```python
from build123d import *

# Parameters (mm, degrees)
F1_DEPTH = 3.175
F2_R     = 5.08
F3_R     = 5.08


with BuildPart() as f1:
    # F0 (on Front) → F1 (new body)
    with BuildSketch(Plane.XZ):
        with BuildLine():
            Line((-6.35, 0), (0, 0))
            Line((0, 0), (0, 22.86))
            Line((0, 22.86), (-6.35, 22.86))
            Line((-6.35, 22.86), (-6.35, 19.685))
            ThreePointArc((-6.35, 19.685), (-4.104936, 18.755064), (-3.175, 16.51))
            ThreePointArc((-3.175, 16.51), (-4.104936, 14.264936), (-6.35, 13.335))
            Line((-6.35, 13.335), (-6.35, 0))
        make_face()
        with BuildLine():
            Line((-12.7, 0), (-6.35, 0))
            Line((-6.35, 0), (-6.35, 13.335))
            ThreePointArc((-6.35, 13.335), (-9.525, 16.51), (-6.35, 19.685))
            Line((-6.35, 19.685), (-6.35, 22.86))
            Line((-6.35, 22.86), (-12.7, 22.86))
            Line((-12.7, 22.86), (-12.7, 0))
        make_face()
    extrude(amount=F1_DEPTH)

    # F2
    f2_edges = [f1.edges().sort_by_distance(p)[0] for p in [
        (0, -1.5875, 22.86),
    ]]
    fillet(f2_edges, radius=F2_R)

    # F3
    f3_edges = [f1.edges().sort_by_distance(p)[0] for p in [
        (-12.7, -1.5875, 22.86),
    ]]
    fillet(f3_edges, radius=F3_R)


solid = f1.part
```
CAD build for the part. Positions are in the model's coordinates, mm. Give positions to 0.01 mm unless a question says otherwise; leave off trailing zeros. Order: outer loops, then holes, each group sorted by start corner. A loop starts at its lowest first (then second) coordinate and runs counter-clockwise, first axis right, second up.
(1) Saw through at B-B, the plane x = -5.75. Give the cut face in (y, z) (3 decimals), then the cut area to 3 significant figures.
(2) Saw through at A-A, the plane y = -0.9. Give the cut face in (x, z) (3 decimals), then the cut area to 3 significant figures.
(3) Drill centre lines: L1, parallel to X at y = -0.85, z = 16.5; L2, parallel to Z at x = -8, y = -2.75; L3, parallel to Z at x = -4.75, y = -0.3. Where is each one in solid material? Low to high.
(4) Saw through at C-C, the plane z = 17.25. Give the cut face in (x, y) (3 decimals).
Results found:
1. outline: (-3.175, 0) - (0, 0) - (0, 13.392) - (-3.175, 13.392) - close; (-3.175, 19.628) - (0, 19.628) - (0, 22.86) - (-3.175, 22.86) - close
1. area: 52.8 mm2
2. outline: (-12.7, 0) - (0, 0) - (0, 17.78) arc R5.08 ccw to (-5.08, 22.86) - (-7.62, 22.86) arc R5.08 ccw to (-12.7, 17.78) - close; hole circle Ø6.35 at (-6.35, 16.51)
2. area: 248 mm2
3. L1: x = -12.7 to -9.52, -3.18 to 0
3. L2: z = 0 to 13.8, 19.22 to 22.85
3. L3: z = 0 to 13.77, 19.25 to 22.85
4. outline: (-12.7, -3.175) - (-9.438, -3.175) - (-9.438, 0) - (-12.7, 0) - close; (-3.262, -3.175) - (0, -3.175) - (0, 0) - (-3.262, 0) - close
